from build123d import *

# Parameters (mm, degrees)
SKETCH2_R               = 4
BOSS_EXTRUDE1_DEPTH     = 2.9
SKETCH3_R               = 3
SKETCH3_R_2             = 1.2
BOSS_EXTRUDE2_DEPTH     = 2
BOSS_EXTRUDE3_START     = 3.4
SKETCH5_R               = 4
SKETCH5_R_2             = 2.1
BOSS_EXTRUDE3_DEPTH     = 3.4
CUT_EXTRUDE1_DEPTH      = 14.494690563
CUT_EXTRUDE1_DEPTH_BACK = 14.494690563
SKETCH7_R               = 0.75


with BuildPart() as part:
    # Sketch2 → Boss-Extrude1 (new body)
    with BuildSketch(Plane.XY):
        with Locations((0, 5.45)):
            Circle(SKETCH2_R)
        Polygon((-0.367620993, 7.7710676), (0.006506124, 8.0210676), (0.367620993, 7.7710676), (0.800691274, 7.893220092), (1.066877674, 7.543865332), (1.516499183, 7.526213179), (1.661700936, 7.111700936), (2.083861586, 6.955972053), (2.093865332, 6.516877674), (2.447241098, 6.238315891), (2.3210676, 5.817620993), (2.5710676, 5.443493876), (2.3210676, 5.082379007), (2.443220092, 4.649308726), (2.093865332, 4.383122326), (2.076213179, 3.933500817), (1.661700936, 3.788299064), (1.505972053, 3.366138414), (1.066877674, 3.356134668), (0.788315891, 3.002758902), (0.367620993, 3.1289324), (-0.006506124, 2.8789324), (-0.367620993, 3.1289324), (-0.800691274, 3.006779908), (-1.066877674, 3.356134668), (-1.516499183, 3.373786821), (-1.661700936, 3.788299064), (-2.083861586, 3.944027947), (-2.093865332, 4.383122326), (-2.447241098, 4.661684109), (-2.3210676, 5.082379007), (-2.5710676, 5.456506124), (-2.3210676, 5.817620993), (-2.443220092, 6.250691274), (-2.093865332, 6.516877674), (-2.076213179, 6.966499183), (-1.661700936, 7.111700936), (-1.505972053, 7.533861586), (-1.066877674, 7.543865332), (-0.788315891, 7.897241098), align=None, mode=Mode.SUBTRACT)
    extrude(amount=-BOSS_EXTRUDE1_DEPTH)

    # Sketch3 → Boss-Extrude2 (add)
    with BuildSketch(Plane.XY):
        with Locations((0, 5.45)):
            Circle(SKETCH3_R)
        with Locations((0, 5.45)):
            Circle(SKETCH3_R_2, mode=Mode.SUBTRACT)
    extrude(amount=BOSS_EXTRUDE2_DEPTH)



with BuildPart() as body_2:
    # Sketch4 → Revolve1 (revolve)
    with BuildSketch(Plane(origin=(-0.84207131, 5.316629007, 0), x_dir=(0.9876883405951381, 0.1564344650402286, 0), z_dir=(-0.1564344650402286, 0.9876883405951381, 0)), mode=Mode.PRIVATE) as revolve1_sk:
        with BuildLine():
            Line((-3.147432166, 1.6), (-7.147432166, 1.6))
            ThreePointArc((-7.147432166, 1.6), (-7.378402049, 1.445670858), (-7.324208861, 1.173223305))
            Line((-7.324208861, 1.173223305), (-4.604538947, -1.546446609))
            ThreePointArc((-4.604538947, -1.546446609), (-4.458092337, -1.9), (-4.604538947, -2.253553391))
            Line((-4.604538947, -2.253553391), (-7.324208861, -4.973223305))
            ThreePointArc((-7.324208861, -4.973223305), (-7.378402049, -5.245670858), (-7.147432166, -5.4))
            Line((-7.147432166, -5.4), (-3.147432166, -5.4))
            Line((-3.147432166, -5.4), (-3.147432166, 1.6))
        make_face()
    revolve(revolve1_sk.sketch.rotate(Axis((0, 5.45, 2), (0, 0, -1)), 189), axis=Axis((0, 5.45, 2), (0, 0, -1)))


with BuildPart() as part_1:
    add(part.part)

    add(body_2.part)  # Boss-Extrude3 merges body 2
    # Sketch5 → Boss-Extrude3 (add)
    with BuildSketch(Plane.XY.offset(2).offset(BOSS_EXTRUDE3_START)):
        with Locations((0, 5.45)):
            Circle(SKETCH5_R)
        with Locations(Location((0, 5.45, 0), (0, 0, 180))):
            Circle(SKETCH5_R_2, mode=Mode.SUBTRACT)
    extrude(amount=-BOSS_EXTRUDE3_DEPTH)

    # Sketch7 → Cut-Extrude1 (cut, two sides: drawn at the far end of the back side and taken through both)
    with BuildSketch(Plane(origin=(-0.84207131, 5.316629007, 0), x_dir=(0.9876883405951381, 0.1564344650402286, 0), z_dir=(-0.1564344650402286, 0.9876883405951381, 0)).offset(-CUT_EXTRUDE1_DEPTH_BACK)):
        with Locations(Location((0.852567834, -1.9, 0), (0, 0, 187.662255661))):
            Circle(SKETCH7_R)
    extrude(amount=CUT_EXTRUDE1_DEPTH + CUT_EXTRUDE1_DEPTH_BACK, mode=Mode.SUBTRACT)


solid = part_1.part
The listing builds one solid part. Answer for the finished solid, in the listing's coordinates (mm). A direction names the side the tool comes from. Give positions to 0.01 mm unless a question says otherwise; leave off trailing zeros. Write each loop counter-clockwise with the first axis right and the second up, starting at its lowest first coordinate (ties: lowest second). Pieces come first, ordered by that corner, then holes.
Item 1: Section C-C, the plane z = 4.5 is taken. Write down the section's boundary in (x, y).
Item 2: Section A-A, the plane z = 0.5 is taken. Write down the section's boundary in (x, y).
Item 3: Determine the mould class of faces 6 (the cylindrical face through (-0.332, 8.8, 2.624)), 7 (the flat face through (3, 6, -2.9)), 8 (the flat face through (1.4, 5.6, 2)) for opening direction Z: released by +Z, released by -Z, zero draft, split by the parting line, or undercut.
Item 4: Which of the six approach directions +Z, -Z, +X, -X, +Y, -Y give full straight-line access (tool end or side, diameter ignored) to faces 1 (the flat face through (-1.2, 6.1, 0)), 2 (the cylindrical face through (-0.65, 2.52, 0.99)), 3 (the cylindrical face through (0.46, 7.5, 3.72)), 4 (the flat face through (2, 4, 5.4)), 5 (the cylindrical face through (0.65, 6.46, 0.99))?
Item 5: Find the intervals of material crossed by line 1 along Z through (x, y) = (-2, 2.25); line 2 along Y through (x, z) = (-1.5, 1); line 3 along X through (y, z) = (5.45, 0.5), in increasing order.
Item 6: Section B-B, the plane z = 3.25 is taken. Write down the section's boundary in (x, y), plus the area to 3 significant figures.
Item 7: Flat-ended cylindrical pins translate along their axes: P1, Ø2, axis at y = -0.5, z = -1.5, coming from the +X side; P2, Ø3.5, axis at x = 0, y = 5.45, coming from the +Z side; P3, Ø2, axis at y = 10.5, z = 1.5, coming from the -X side. Find the tip coordinate at first contact, or state that the pin passes through.
Completed:
1. outline: circle Ø15.41 at (0, 5.45); hole circle Ø4.2 at (0, 5.45)
2. outline: circle Ø13.01 at (0, 5.45); circle Ø6 at (0, 5.45); hole circle Ø8 at (0, 5.45); hole circle Ø2.4 at (0, 5.45)
3. face 6: undercut
3. face 7: released by -Z
3. face 8: released by +Z
4. face 1: -Z
4. face 2: none
4. face 3: +Z
4. face 4: +Z, +X, -X, +Y, -Y
4. face 5: +Z, -Z
5. line 1: z = -2.9 to 0, 2 to 5.4
5. line 2: y = -0.36 to 1.74, 2.85 to 8.05, 9.16 to 11.26
5. line 3: x = -6.5 to -4, -3 to -1.2, 1.2 to 3, 4 to 6.5
6. outline: circle Ø12.91 at (0, 5.45); hole circle Ø4.2 at (0, 5.45)
6. area: 117 mm2
7. P1: stops at x = 6.59
7. P2: stops at z = 2
7. P3: stops at x = -4.47
